```python
from build123d import *

# Parameters (mm, degrees)
F0_R     = 13
F1_DEPTH = 0.3
F2_R     = 1
F3_DEPTH = 0.5


with BuildPart() as f1:
    # F0 (on Top) → F1 (new body)
    with BuildSketch(Plane.XY):
        Circle(F0_R)
    extrude(amount=F1_DEPTH)

    # F2 (on face) → F3 (join)
    with BuildSketch(Plane.XY.offset(0.3)):
        with BuildLine():
            Line((6.5, 1.5), (6.5, 6.5))
            Line((6.5, 6.5), (1.5, 6.5))
            ThreePointArc((1.5, 6.5), (0, 5), (-1.5, 6.5))
            Line((-1.5, 6.5), (-6.5, 6.5))
            Line((-6.5, 6.5), (-6.5, 1.5))
            ThreePointArc((-6.5, 1.5), (-5, 0), (-6.5, -1.5))
            Line((-6.5, -1.5), (-6.5, -6.5))
            Line((-6.5, -6.5), (-1.5, -6.5))
            ThreePointArc((-1.5, -6.5), (0, -5), (1.5, -6.5))
            Line((1.5, -6.5), (6.5, -6.5))
            Line((6.5, -6.5), (6.5, -1.5))
            ThreePointArc((6.5, -1.5), (5, 0), (6.5, 1.5))
        make_face()
        Circle(F2_R, mode=Mode.SUBTRACT)
    extrude(amount=F3_DEPTH)


solid = f1.part
```
CAD build for the part. Positions are in the model's coordinates, mm. A direction names the side the tool comes from. Round coordinates to 2 decimals unless told otherwise and drop trailing zeros. Order: outer loops, then holes, each group sorted by start corner. A loop starts at its lowest first (then second) coordinate and runs counter-clockwise, first axis right, second up.
Item 1: Mould opens along X. For faces 5 (the face through (5, 0, 0.5)), 6 (the face through (0, 0, 0.3)), 7 (the face through (-5, 0, 0.5)) say: pulls with the +X half, pulls with the -X half, needs draft (parallel to the pull), parting line crosses it, or undercut.
Item 2: Saw through at A-A on z = 0.6. Write the cut outline in (x, y), then the cut area to 3 significant figures.
Item 3: Probe line 1 along Y through (x, z) = (0, 0.4); line 2 along X through (y, z) = (-0.25, 0.1); line 3 along Z through (x, y) = (-3.25, -11.5). List the from-to ranges inside material, lowest first.
Item 4: Tool access for faces 1 (the face through (-0.217, -0.976, 0.546)), 2 (the face through (0, 0, 0)), 3 (the face through (0, -5, 0.5)), 4 (the face through (0, 5, 0.5)): list every direction of +Z, -Z, +X, -X, +Y, -Y with a clear straight run to the whole face (end or side of a thin tool).
Item 5: Saw through at B-B on x = 0. Write the cut outline in (y, z), then the cut area to 3 significant figures.
Item 6: Saw through at D-D on y = 8.75. Write the cut outline in (x, z), then the cut area to 3 significant figures.
Reported:
1. face 5: pulls with the +X half
1. face 6: undercut
1. face 7: pulls with the -X half
2. outline: (-6.5, -6.5) - (-1.5, -6.5) arc R1.5 cw to (1.5, -6.5) - (6.5, -6.5) - (6.5, -1.5) arc R1.5 cw to (6.5, 1.5) - (6.5, 6.5) - (1.5, 6.5) arc R1.5 cw to (-1.5, 6.5) - (-6.5, 6.5) - (-6.5, 1.5) arc R1.5 cw to (-6.5, -1.5) - close; hole circle Ø2 at (0, 0)
2. area: 152 mm2
3. line 1: y = -5 to -1, 1 to 5
3. line 2: x = -13 to 13
3. line 3: z = 0 to 0.3
4. face 1: +Z
4. face 2: -Z, +X, -X, +Y, -Y
4. face 3: +Z, -Y
4. face 4: +Z, +Y
5. outline: (-13, 0) - (13, 0) - (13, 0.3) - (5, 0.3) - (5, 0.8) - (1, 0.8) - (1, 0.3) - (-1, 0.3) - (-1, 0.8) - (-5, 0.8) - (-5, 0.3) - (-13, 0.3) - close
5. area: 11.8 mm2
6. outline: (-9.61, 0) - (9.61, 0) - (9.61, 0.3) - (-9.61, 0.3) - close
6. area: 5.77 mm2
